```python
from build123d import *

# Parameters (mm, degrees)
F1_W    = 23.5887104645
F1_H    = 20.866939798
F1_W_2  = 22.3185494542
F1_H_2  = 13.6088710278
F1_W_3  = 19.2338721827
F3_SIZE = 5


# Not quite as in the source:
# - a fillet or chamfer that OpenCascade refuses, or shapes differently, is made with other operations: its cross-section is extruded or revolved along the edge and cut away or added


with BuildPart() as f2:
    # F1 (on Front) → F2 (revolve)
    with BuildSketch(Plane.XZ):
        Polygon((-13.9717748389, 54.798386991), (-70.7661360502, 54.798386991), (-70.7661360502, 17.7822578698), (-37.5604853034, 17.7822578698), (-37.5604853034, 38.6491976678), (-13.9717748389, 38.6491976678), align=None)
        Polygon((15.2419358492, 38.6491976678), (-13.9717748389, 38.6491976678), (-13.9717748389, 17.7822578698), (-37.5604853034, 17.7822578698), (-37.5604853034, 17.6008082926), (-3.9919363335, 17.6008082926), (-3.9919363335, 31.2096793205), (15.2419358492, 31.2096793205), align=None)
        with Locations((-25.7661300711, 28.2157277688)):
            Rectangle(F1_W, F1_H)
        with Locations((26.4012105763, 24.4052438065)):
            Rectangle(F1_W_2, F1_H_2)
        with Locations((5.6249997579, 24.4052438065)):
            Rectangle(F1_W_3, F1_H_2)
    revolve(axis=Axis((0.2721734345, 0, 0), (1, 0, 0)))

    # F3
    f3_edges = [f2.edges().sort_by_distance(p)[0] for p in [
        (-13.971775, 0, -54.798387),
        (-70.766136, 0, -54.798387),
        (-42.368955, 0, 54.798387),
        (37.560485, 0, -17.600808),
    ]]
    chamfer(f3_edges, length=F3_SIZE)

    # F4: chamfer of 5 on 5 edges, made by hand

    # F4_s1 → F4_t2 (revolve)
    with BuildSketch(Plane.XZ):
        Polygon((-13.9717748389, 43.6491976678), (-8.9717748389, 38.6491976678), (-13.9717748389, 38.6491976678), align=None)
    revolve(axis=Axis((-13.9717748389, 0, 0), (1, 0, 0)))

    # F4_s3 → F4_t4 (revolve, cut)
    with BuildSketch(Plane.XZ):
        Polygon((32.5604853034, 31.2096793205), (37.5604853034, 26.2096793205), (37.5604853034, 31.2096793205), align=None)
    revolve(axis=Axis((37.5604853034, 0, 0), (1, 0, 0)), mode=Mode.SUBTRACT)

    # F4_s5 → F4_t6 (revolve, cut)
    with BuildSketch(Plane.XZ):
        Polygon((36.0960192093, 21.1363421986), (37.5604853034, 24.6718761045), (37.5604853034, 22.6008082926), align=None)
    revolve(axis=Axis((37.5604853034, 0, 0), (1, 0, 0)), mode=Mode.SUBTRACT)

    # F4_s7 → F4_t8 (revolve, cut)
    with BuildSketch(Plane.XZ):
        Polygon((10.2419358492, 38.6491976678), (15.2419358492, 33.6491976678), (15.2419358492, 38.6491976678), align=None)
    revolve(axis=Axis((15.2419358492, 0, 0), (1, 0, 0)), mode=Mode.SUBTRACT)


solid = f2.part
```
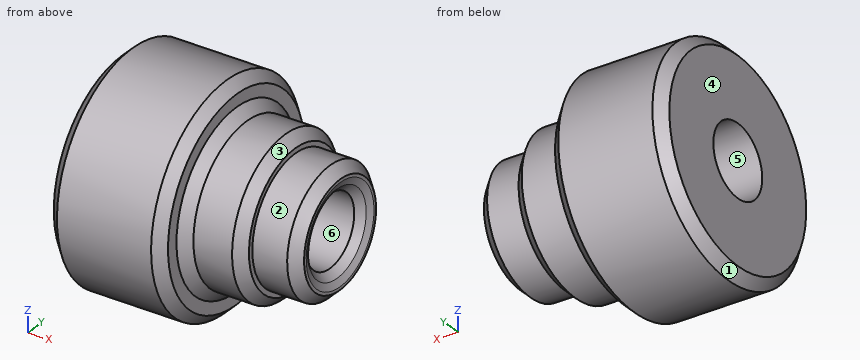
Check sheet for the modelled part. Datum: model origin and axes. Units: mm. Face numbers are marked on the shaded views. A direction names the side the tool comes from. Give positions to 0.01 mm unless a question says otherwise; leave off trailing zeros. Write each loop counter-clockwise with the first axis right and the second up, starting at its lowest first coordinate (ties: lowest second). Pieces come first, ordered by that corner, then holes.
Item 1: Scan lines: L1, parallel to Y at x = 18, z = 0; L2, parallel to Z at x = -60.5, y = 0. Record each from-to range of solid material in increasing order.
Item 2: Access from +Z, -Z, +X, -X, +Y, -Y to the whole of each face (thin tool, end or side, straight path). Record for the marked faces 1 and 2.
Item 3: Cross-section at D-D (x = 7.5). Enter the section's corners in (y, z).
Item 4: Gauge pin test, flat ends, axial feed: pin 1 (12 mm diameter, centred on y = -26, z = 33, fed in from +X); pin 2 (8 mm diameter, centred on x = -2.5, y = -3.5, fed in from -Z); pin 3 (4 mm diameter, centred on x = 15.5, z = -10, fed in from -Y). Record the tip position at first contact, or that the pin passes through.
Item 5: Cross-section at C-C (x = -20.5). Enter the section's corners in (y, z), and give its area (3 significant figures).
Item 6: Draft check along Y on the marked faces 3, 4, 5 and 6. Enter one of: released by +Y, released by -Y, zero draft, split by the parting line, or undercut.
Report:
1. L1: y = -31.21 to -17.6, 17.6 to 31.21
1. L2: z = -54.8 to -17.78, 17.78 to 54.8
2. face 1: -X
2. face 2: +X
3. outline: circle Ø77.3 at (0, 0); hole circle Ø35.2 at (0, 0)
4. pin 1: stops at x = 12.88
4. pin 2: stops at z = -38.65
4. pin 3: stops at y = -34.03
5. outline: circle Ø109.6 at (0, 0); hole circle Ø35.2 at (0, 0)
5. area: 8,460 mm2
6. face 3: split by the parting line
6. face 4: zero draft
6. face 5: undercut
6. face 6: undercut
